Read the model definition and answer for the solid it produces. Units are mm, in the model's axes. A direction names the side the tool comes from. Give positions to 0.01 mm unless a question says otherwise; leave off trailing zeros. Write each loop counter-clockwise with the first axis right and the second up, starting at its lowest first coordinate (ties: lowest second). Pieces come first, ordered by that corner, then holes. Notation, with made-up numbers: M 53.5,8 L 98.5,8 A12 cw 98.5,26 Z; hole C 28,57.25 d5. An arc over 180 degrees is marked long. Use a Markdown table: item, result. Add a question column.
Item 1: A cutting plane is placed at B-B on y = -30. Determine the outline of the cut face in (x, z).
Item 2: Consider probe 1 along Z at (x, y) = (0, -34); probe 2 along X at (y, z) = (-8.5, 7.5). Determine where each line is inside the solid, lowest interval first. Write a range as [from, to].
Item 3: For faces 1 (the flat face through (46, -19, -17.321)), 2 (the flat face through (42, 0, 2)), determine the directions among +Z, -Z, +X, -X, +Y, -Y from which every point of the face is accessible in a straight line to the end or side of a thin tool.
Item 4: A cutting plane is placed at A-A on x = 0. Determine the outline of the cut face in (y, z).
Item 5: The mould has two halves that part along Z. Classify faces 3 (the flat face through (54, -15, 8)), 4 (the cylindrical face through (30.121, -7.395, 14.444)), 5 (the cylindrical face through (72.502, -7.395, 17.683)): pulls with the +Z half, pulls with the -Z half, needs draft (parallel to the pull), parting line crosses it, or undercut.
Item 6: A cutting plane is placed at C-C on y = -12. Determine the outline of the cut face in (x, z) (1 decimal), then the cut area to 3 significant figures.
Item 7: Given P1, Ø2, axis at x = 52.5, y = -9, coming from the -Z side; P2, Ø18, axis at x = 0, z = 0, coming from the +Y side; P3, Ø1.5, axis at y = -41, z = 5.5, coming from the +X side; P4, Ø6, axis at y = -31, z = 14, coming from the -X side, each flat-ended and moving along its own axis, determine where each tip first touches the part or whether it passes through.
Item 8: A cutting plane is placed at D-D on z = -13. Determine the outline of the cut face in (x, y).
from build123d import *
from build123d import SkipClean  # not in build123d's __all__

# Parameters (mm, degrees)
F0_R     = 10
F1_DEPTH = 15
F2_R     = 10
F3_DEPTH = 35
F5_DEPTH = 35
F7_DEPTH = 15


# Not quite as in the source:
# - after a boolean that leaves OpenCascade's solid faulty, fix() repairs it


with BuildPart() as f1:
    # F0 (on Front) → F1 (new body)
    with BuildSketch(Plane.XZ):
        with BuildLine():
            ThreePointArc((46.3350602938, 25.7917141365), (29.8412578998, 14.3770862565), (10, 17.3205080757))
            ThreePointArc((10, 17.3205080757), (-20, 0), (10, -17.3205080757))
            Line((10, -17.3205080757), (82.9639062402, -17.3205080757))
            Line((82.9639062402, -17.3205080757), (82.9639062402, 14.6794919243))
            ThreePointArc((82.9639062402, 14.6794919243), (68.7700702523, 33.818155918), (46.3350602938, 25.7917141365))
        make_face()
        with BuildLine():
            ThreePointArc((5, 8.6602540378), (8.6602540378, 5), (10, 0))
            ThreePointArc((10, 0), (-8.6602540378, -5), (5, 8.6602540378))
        make_face(mode=Mode.SUBTRACT)
        with Locations((62.9639062402, 14.6794919243)):
            Circle(F0_R, mode=Mode.SUBTRACT)
    extrude(amount=F1_DEPTH)

    # F2 (on face) → F3 (join)
    with BuildSketch(Plane.XZ.offset(15)):
        with BuildLine():
            ThreePointArc((10, -17.3205080757), (17.3205080757, -10), (20, 0))
            ThreePointArc((20, 0), (17.3205080757, 10), (10, 17.3205080757))
            ThreePointArc((10, 17.3205080757), (-20, 0), (10, -17.3205080757))
        make_face()
        Circle(F2_R, mode=Mode.SUBTRACT)
    with SkipClean():  # cleaning this boolean's faces spoils the solid; the shape is the same uncleaned
        extrude(amount=F3_DEPTH)

    # F4 (on face) → F5 (join)
    with BuildSketch(Plane.XZ.offset(15)):
        with BuildLine():
            Line((10, -17.3205080757), (82.9639062402, -17.3205080757))
            Line((82.9639062402, -17.3205080757), (82.9639062402, -2.3205080757))
            Line((82.9639062402, -2.3205080757), (19.8649249249, -2.3205080757))
            ThreePointArc((19.8649249249, -2.3205080757), (16.710129718, -10.9896116769), (10, -17.3205080757))
        make_face()
    extrude(amount=F5_DEPTH)

    add(f1.part.fix(), mode=Mode.REPLACE)

    # F6 (on face) → F7 (cut, through all)
    with BuildSketch(Plane.XY.offset(-2.3205080757)):
        Polygon((82.9639062402, -50), (82.9639062402, -25), (32.9639062402, -50), align=None)
    extrude(amount=-F7_DEPTH, mode=Mode.SUBTRACT)


solid = f1.part
Filled in:
| question | item | result |
|---|---|---|
| 1 | outline | M 10,-17.32 L 72.96,-17.32 L 72.96,-2.32 L 19.86,-2.32 A20 ccw long Z; hole C 0,0 d20 |
| 2 | probe 1 | [-20, -10], [10, 20] |
| 2 | probe 2 | [-18.54, -6.61], [6.61, 56], [69.92, 82.96] |
| 3 | face 1 | -Z, +X, +Y, -Y |
| 3 | face 2 | +Z, -Z, +X, -X, +Y |
| 4 | outline | M -50,-20 L 0,-20 L 0,-10 L -50,-10 Z; M -50,10 L 0,10 L 0,20 L -50,20 Z |
| 5 | face 3 | needs draft |
| 5 | face 4 | pulls with the +Z half |
| 5 | face 5 | undercut |
| 6 | outline | M 10,-17.3 L 83,-17.3 L 83,14.7 A20 ccw 46.3,25.8 A27.3 cw 10,17.3 A20 ccw long Z; hole C 0,0 d20; hole C 63,14.7 d20 |
| 6 | area | 3,380 mm² |
| 7 | P1 | z = -17.32 |
| 7 | P2 | through |
| 7 | P3 | x = 19.43 |
| 7 | P4 | x = -16.7 |
| 8 | outline | M -15.2,-50 L 32.96,-50 L 82.96,-25 L 82.96,0 L -15.2,0 Z |
